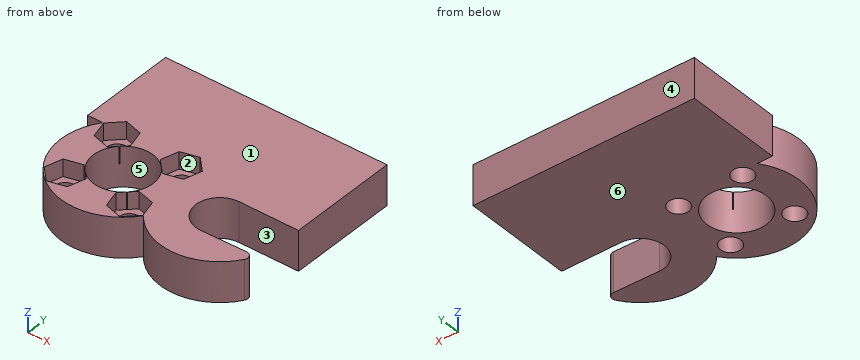
from build123d import *

# Parameters (mm, degrees)
F0_R     = 1.8
F0_R_2   = 5.25
F1_DEPTH = 7
F3_DEPTH = 3


# Not quite as in the source:
# - a feature names something its author has since deleted; it is built from what else it names


with BuildPart() as f1:
    # F0 (on Top) → F1 (new body)
    with BuildSketch(Plane.XY):
        with BuildLine():
            ThreePointArc((17, -4.2), (12.8000000278, 0.000483474), (17.000966948, 4.1999998887))
            Line((17.000966948, 4.1999998887), (27.4750051144, 4.1999998887))
            Line((27.4750051144, 4.1999998887), (27.4750051144, 23.499993239))
            Line((27.4750051144, 23.499993239), (-11.5249948856, 23.5))
            Line((-11.5249948856, 23.5), (-11.5249978328, 6.5))
            Line((-11.5249978328, 6.5), (-8.8741196746, 6.5))
            ThreePointArc((-8.8741196746, 6.5), (-6.5288626997, -8.8529064068), (8.8315992647, -6.5576561688))
            ThreePointArc((8.8315992647, -6.5576561688), (17.5981324789, -10.4579090901), (25.8628092229, -5.5835685434))
            ThreePointArc((25.8628092229, -5.5835685434), (25.8873322976, -4.5593941021), (24.9978561691, -4.051096075))
            Line((24.9978561691, -4.051096075), (17, -4.2))
        make_face()
        with Locations((-5.6568542495, -5.6568542495)):
            Circle(F0_R, mode=Mode.SUBTRACT)
        with Locations((5.6568542495, -5.6568542495)):
            Circle(F0_R, mode=Mode.SUBTRACT)
        with Locations((-5.6568542495, 5.6568542495)):
            Circle(F0_R, mode=Mode.SUBTRACT)
        Circle(F0_R_2, mode=Mode.SUBTRACT)
        with Locations((5.6568542495, 5.6568542495)):
            Circle(F0_R, mode=Mode.SUBTRACT)
    extrude(amount=-F1_DEPTH)

    # F2 (on face) → F3 (cut)
    with BuildSketch(Plane.XY):
        Polygon((-7.8783541444, -3.3878739609), (-8.7325987676, -6.4462394487), (-6.5110988727, -8.7152197373), (-3.4353543546, -7.9258345381), (-2.5811097314, -4.8674690503), (-4.8026096263, -2.5984887617), align=None)
        Polygon((3.3878739609, -7.8783541444), (6.4462394487, -8.7325987676), (8.7152197373, -6.5110988727), (7.9258345381, -3.4353543546), (4.8674690503, -2.5811097314), (2.5984887617, -4.8026096263), align=None)
        Polygon((7.8783541444, 3.3878739609), (8.7325987676, 6.4462394487), (6.5110988727, 8.7152197373), (3.4353543546, 7.9258345381), (2.5811097314, 4.8674690503), (4.8026096263, 2.5984887617), align=None)
        Polygon((-3.3878739609, 7.8783541444), (-6.4462394487, 8.7325987676), (-8.7152197373, 6.5110988727), (-7.9258345381, 3.4353543546), (-4.8674690503, 2.5811097314), (-2.5984887617, 4.8026096263), align=None)
    extrude(amount=-F3_DEPTH, mode=Mode.SUBTRACT)


solid = f1.part
Read the model definition and answer for the solid it produces. Units are mm, in the model's axes. Face numbers are marked on the shaded views. A direction names the side the tool comes from. Give positions to 0.01 mm unless a question says otherwise; leave off trailing zeros. Loops run counter-clockwise (first coordinate to the right, second up) from the corner with the lowest first, then second, coordinate; pieces in that order, holes last. Notation, with made-up numbers: M 5,-15.5 L 13,-15.5 A13 cw 13,-2.5 Z; hole C 28,-15.75 d4. An arc over 180 degrees is marked long. Write each question's results on one line, items separated by ' | '.
1. Straight lines are drawn through the part: line 1 (Y direction, x = 0, z = -6); line 2 (X direction, y = -6, z = -6.5); line 3 (X direction, y = 4.5, z = -4.75) (3 decimals). For each, find the intervals that lie inside material, in ascending order. Write a range as [from, to].
Values:
line 1: y = [-11, -5.25], [5.25, 23.5] | line 2: x = [-9.22, -7.42], [-3.89, 3.89], [7.42, 25.59] | line 3: x = [-10.037, -7.036], [-4.278, -2.704], [2.704, 4.278], [7.036, 27.475]
2. Section B-B on y = -0.5 is taken. Give the vertices of the cut face in (x, z), plus the area to 3 significant figures.
Values:
outline: M -10.99,-7 L -5.23,-7 L -5.23,0 L -10.99,0 Z; M 5.23,-7 L 12.83,-7 L 12.83,0 L 5.23,0 Z | area: 93.6 mm^2
3. A tool of negligible diameter and unlimited length cuts with its end or side. For the marked faces 1, 2 and 3, from which of +Z, -Z, +X, -X, +Y, -Y can it reach the whole face along a straight path? Write none if from no direction.
Values:
face 1: +Z, +X, -X, +Y, -Y | face 2: +Z | face 3: +Z, -Z, +X
4. Section A-A on x = 0 is taken. Give the vertices of the cut face in (y, z).
Values:
outline: M -11,-7 L -5.25,-7 L -5.25,0 L -11,0 Z; M 5.25,-7 L 23.5,-7 L 23.5,0 L 5.25,0 Z
5. The mould has two halves that part along Y. Classify the marked faces 4, 5 and 6: pulls with the +Y half, pulls with the -Y half, needs draft (parallel to the pull), parting line crosses it, or undercut.
Values:
face 4: pulls with the +Y half | face 5: undercut | face 6: needs draft
6. Given pin 1 (3 mm diameter, centred on x = 5.5, y = 6.5, fed in from +Z); pin 2 (2 mm diameter, centred on x = -11, z = -4.5, fed in from -Y); pin 3 (3.5 mm diameter, centred on x = 21.5, z = -4, fed in from -Y), each flat-ended and moving along its own axis, determine where each tip first touches the part or whether it passes through.
Values:
pin 1: stops at z = -3 | pin 2: stops at y = -4.58 | pin 3: stops at y = -10.11
7. Section C-C on z = -5 is taken. Give the vertices of the cut face in (x, y) (3 decimals).
Values:
outline: M -11.525,6.5 L -8.874,6.5 A11 ccw 8.832,-6.558 A10.475 ccw 25.863,-5.584 A1 ccw 24.998,-4.051 L 17,-4.2 A4.2 cw 17.001,4.2 L 27.475,4.2 L 27.475,23.5 L -11.525,23.5 Z; hole C -5.657,-5.657 d3.6; hole C -5.657,5.657 d3.6; hole C 0,0 d10.5; hole C 5.657,-5.657 d3.6; hole C 5.657,5.657 d3.6
